from build123d import *

# Parameters (mm, degrees)
CUT_EXTRUDE_1_DEPTH      = 3
CUT_EXTRUDE_1_DEPTH_BACK = 3


with BuildPart() as part:
    # Sketch 1 → Revolve 1 (revolve)
    with BuildSketch(Plane.XY, mode=Mode.PRIVATE) as revolve_1_sk:
        with BuildLine():
            Line((0, 25.8), (3, 25.8))
            ThreePointArc((3, 25.8), (3.707106781, 25.507106781), (4, 24.8))
            Line((4, 24.8), (4, 9.4))
            Line((4, 9.4), (5, 9.4))
            Line((5, 9.4), (5, 0))
            Line((5, 0), (2.5, 0))
            Line((2.5, 0), (2.5, -19.5095))
            Line((2.5, -19.5095), (2.0095, -20))
            Line((2.0095, -20), (0, -20))
            Line((0, -20), (0, 25.8))
        make_face()
    revolve(revolve_1_sk.sketch.rotate(Axis((0, -20, 0), (0, 1, 0)), 270), axis=Axis((0, -20, 0), (0, 1, 0)))

    # Sketch 2 → Cut-Extrude 1 (cut, two sides: drawn at the far end of the back side and taken through both)
    with BuildSketch(Plane(origin=(0, 25.8, 0), x_dir=(1, 0, 0), z_dir=(0, 1, 0)).offset(-CUT_EXTRUDE_1_DEPTH_BACK)):
        Polygon((-1.5, 0.866025404), (-1.5, -0.866025404), (0, -1.732050808), (1.5, -0.866025404), (1.5, 0.866025404), (0, 1.732050808), align=None)
    extrude(amount=CUT_EXTRUDE_1_DEPTH + CUT_EXTRUDE_1_DEPTH_BACK, mode=Mode.SUBTRACT)


solid = part.part
Design review of the part built by this model. Coordinates are the model's own, in mm. A direction names the side the tool comes from. Give positions to 0.01 mm unless a question says otherwise; leave off trailing zeros. Loops run counter-clockwise (first coordinate to the right, second up) from the corner with the lowest first, then second, coordinate; pieces in that order, holes last. Notation, with made-up numbers: (56.5, 41.5) - (88.5, 41.5) arc R19 ccw to (88.5, 50.5) - close; hole circle Ø10 at (58, 6.25). An arc over 180 degrees is marked (long way). Write item = value, one per line.
1) To check wall thickness, follow line 1 (Y direction, x = 0.75, z = 3); line 2 (Y direction, x = -0.25, z = -1.5); line 3 (X direction, y = -12.5, z = 0). State the ranges of each line that lie inside material, in increasing order.
Result sheet:
line_1 = 0 to 25.8
line_2 = -20 to 22.8
line_3 = -2.5 to 2.5
2) Draft analysis for pull direction X (two halves, no side actions). For faces 1 (the face through (0.74, 24.279, 1.305)), 2 (the face through (0, -20, 0)), 3 (the face through (-4.88, 4.63, -1.08)), state which applies: +X half, -X half, draft (parallel to the pull), parting line (faces both ways), or undercut.
Result sheet:
face_1 = undercut
face_2 = draft
face_3 = parting line
3) Take a section at B-B on y = 8. State the section outline as (x, z) points.
Result sheet:
outline = circle Ø10 at (0, 0)
4) Tool access review of faces 4 (the face through (-2, 0, 2)), 5 (the face through (1.5, 24, 0)), 6 (the face through (-1.3, 25.8, -1.3)): name each direction out of +Z, -Z, +X, -X, +Y, -Y from which nothing blocks a thin tool from reaching the whole face with its end or side.
Result sheet:
face_4 = -Y
face_5 = +Y
face_6 = +Z, -Z, +X, -X, +Y
5) Clearance check with flat-ended pins moving along their axes: pin 1 Ø2 at (y, z) = (17.5, -1.5) entering from -X; pin 2 Ø3 at (y, z) = (5, 2.5) entering from -X; pin 3 Ø4 at (x, y) = (-1.5, -4.5) entering from -Z. State where each tip first meets the part, or that it passes through.
Result sheet:
pin_1 = -3.97
pin_2 = -4.9
pin_3 = -2.5
6) Take a section at A-A on z = 0. State the section outline as (x, y) points.
Result sheet:
outline = (-5, 0) - (-2.5, 0) - (-2.5, -19.51) - (-2.01, -20) - (2.01, -20) - (2.5, -19.51) - (2.5, 0) - (5, 0) - (5, 9.4) - (4, 9.4) - (4, 24.8) arc R1 ccw to (3, 25.8) - (1.5, 25.8) - (1.5, 22.8) - (-1.5, 22.8) - (-1.5, 25.8) - (-3, 25.8) arc R1 ccw to (-4, 24.8) - (-4, 9.4) - (-5, 9.4) - close
